Verification items for this drawing (mm, ordinates from the low corner). Round coordinates to 2 decimals unless told otherwise and drop trailing zeros. Loops run counter-clockwise (first coordinate to the right, second up) from the corner with the lowest first, then second, coordinate; pieces in that order, holes last. Notation, with made-up numbers: M 0.25,1 L 48.25,1 A17 cw 48.25,24 Z; hole C 51,56 d3. An arc over 180 degrees is marked long. Write item = value, one per line.
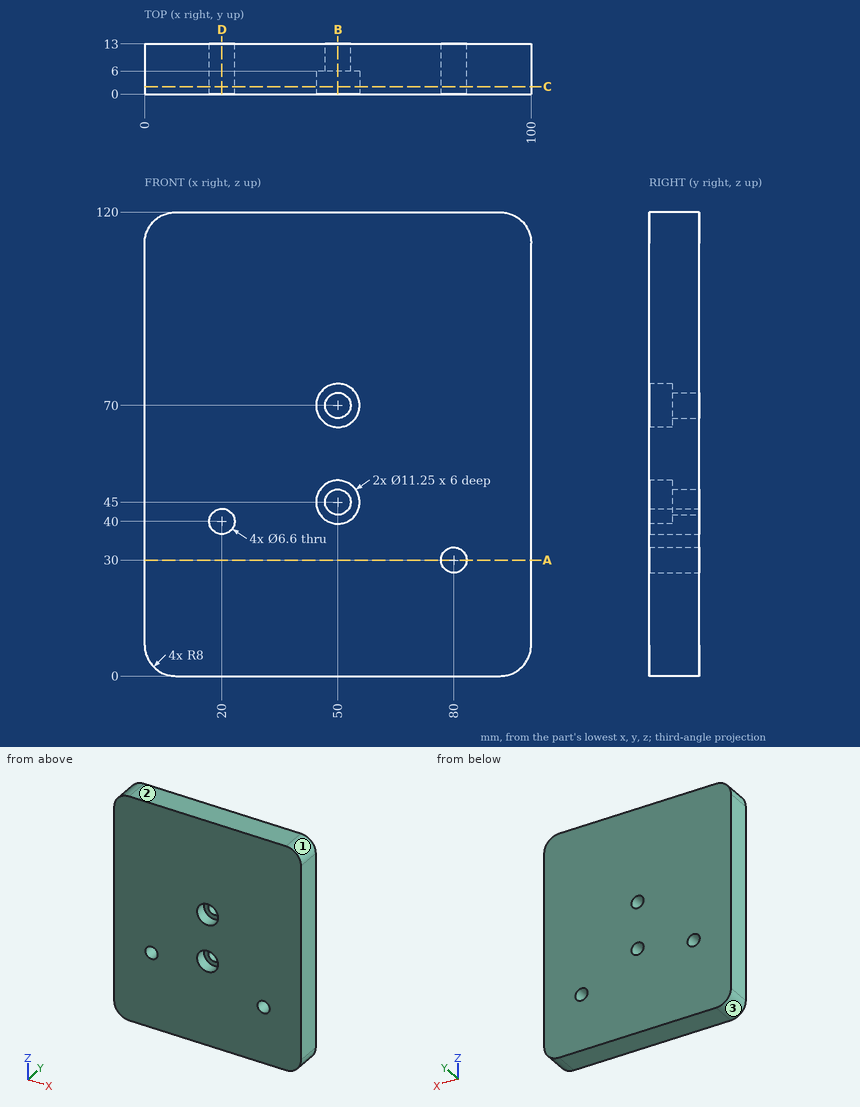
(1) Sectioned sample at C-C on y = 2. Record the cut outline in (x, z) (3 decimals), then the cut area to 3 significant figures.
Result set:
outline = M 0,8 A8 ccw 8,0 L 92,0 A8 ccw 100,8 L 100,112 A8 ccw 92,120 L 8,120 A8 ccw 0,112 Z; hole C 20,40 d6.6; hole C 50,45 d11.25; hole C 50,70 d11.25; hole C 80,30 d6.6
area = 11,700 mm2
(2) Sectioned sample at D-D on x = 20. Record the cut outline in (y, z).
Result set:
outline = M 0,0 L 13,0 L 13,36.7 L 0,36.7 Z; M 0,43.3 L 13,43.3 L 13,120 L 0,120 Z
(3) Sectioned sample at A-A on z = 30. Record the cut outline in (x, y), then the cut area to 3 significant figures.
Result set:
outline = M 0,0 L 76.7,0 L 76.7,13 L 0,13 Z; M 83.3,0 L 100,0 L 100,13 L 83.3,13 Z
area = 1,210 mm2
(4) Sectioned sample at B-B on x = 50. Record the cut outline in (y, z) (3 decimals).
Result set:
outline = M 0,0 L 13,0 L 13,41.7 L 6,41.7 L 6,39.375 L 0,39.375 Z; M 0,50.625 L 6,50.625 L 6,48.3 L 13,48.3 L 13,66.7 L 6,66.7 L 6,64.375 L 0,64.375 Z; M 0,75.625 L 6,75.625 L 6,73.3 L 13,73.3 L 13,120 L 0,120 Z
(5) Depth check by flat-ended pin: pin 1 Ø7.5 at (x, z) = (50, 70) entering from -Y. Enter the tip coordinate at first touch or a pass-through.
Result set:
pin_1 = 6
(6) Material ranges on line 1 along Z through (x, y) = (50, 11.75); line 2 along Z through (x, y) = (50, 4.3) (3 decimals); line 3 along Z through (x, y) = (20, 8.5), recorded low to high. Write a range as from..to.
Result set:
line_1 = 0..41.7, 48.3..66.7, 73.3..120
line_2 = 0..39.375, 50.625..64.375, 75.625..120
line_3 = 0..36.7, 43.3..120
(7) Release check for a two-part mould opening along X. For the marked faces 1, 2 and 3 record: released by +X, released by -X, zero draft, split by the parting line, or undercut.
Result set:
face_1 = released by +X
face_2 = zero draft
face_3 = released by -X
